Study the drawing (mm; zero at the part's minimum x, y, z) and answer. A direction names the side the tool comes from. Round coordinates to 2 decimals unless told otherwise and drop trailing zeros. Write each loop counter-clockwise with the first axis right and the second up, starting at its lowest first coordinate (ties: lowest second). Pieces come first, ordered by that corner, then holes. Notation, with made-up numbers: (66.5, -34.75) - (85.5, -34.75) arc R32 ccw to (85.5, -8.75) - close; hole circle Ø3 at (76.5, 35.5). An arc over 180 degrees is marked (long way). Use one line per item in the form item = value. Start each with the question number.
1) The part is cut by section D-D, the plane y = 35.5. Give the vertices of the cut face in (x, z), plus the area to 3 significant figures.
2) For a pull along Y with two mould halves and no side action, classify the marked faces 1, 2, 3 and 4 as released by +Y, released by -Y, zero draft, split by the parting line, or undercut.
3) The part is cut by section B-B, the plane z = 4.25. Give the vertices of the cut face in (x, y).
4) Each of these flat-tipped pins is pushed along its axis until it touches: pin 1 (1.2 mm diameter, centred on x = 15.5, z = 5, fed in from +Y); pin 2 (3 mm diameter, centred on y = 39, z = 22.5, fed in from +X); pin 3 (1.5 mm diameter, centred on x = 16.5, z = 20.5, fed in from +Y). Where does it stop, or does it pass through?
5) The part is cut by section C-C, the plane x = 11.5. Give the vertices of the cut face in (y, z), plus the area to 3 significant figures.
6) For the marked faces 5, 6, 7, 8 and 9, determine the directions among +Z, -Z, +X, -X, +Y, -Y from which every point of the face is accessible in a straight line to the end or side of a thin tool.
7) Consider line 1 along Y through (x, z) = (11, 3.2); line 2 along Z through (x, y) = (10.75, 23.5); line 3 along X through (y, z) = (26, 1.3). Determine where each line is inside the solid, lowest interval first. Write a range as from..to.
8) The part is cut by section A-A, the plane y = 6. Give the vertices of the cut face in (x, z), plus the area to 3 significant figures.
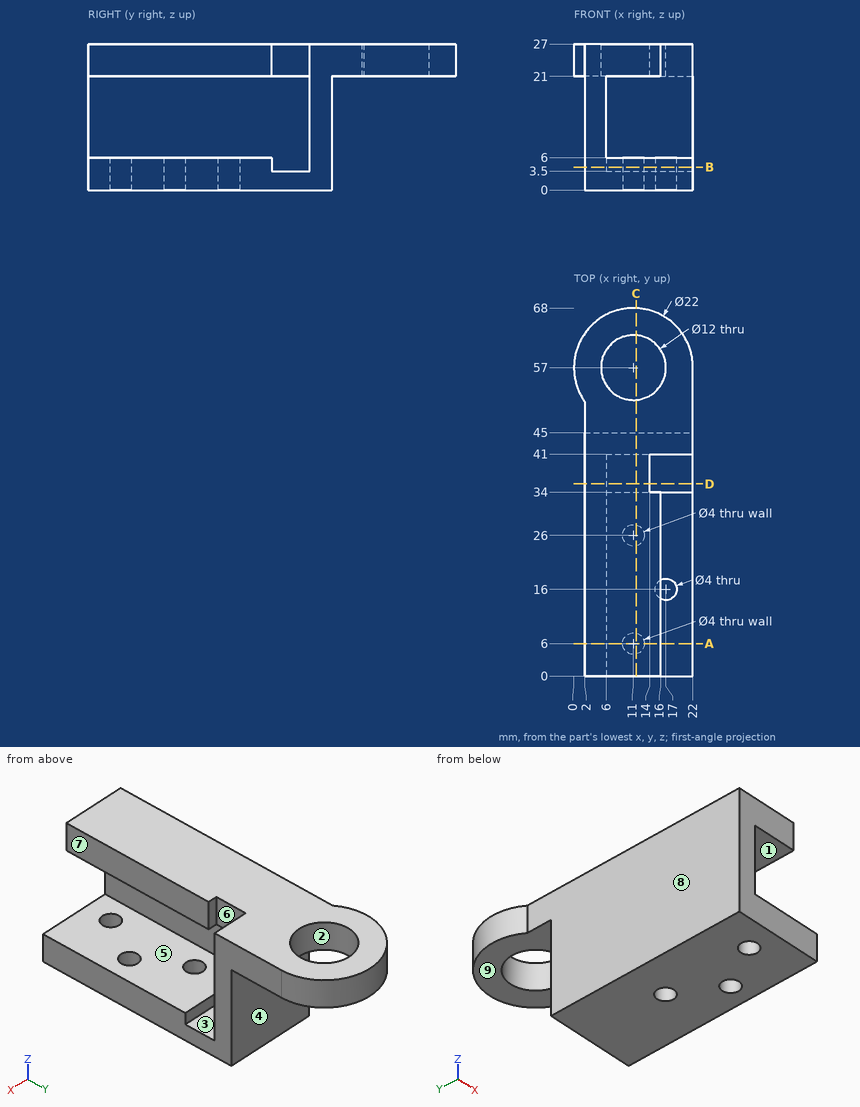
Geometry results:
q1.outline = (2, 0) - (22, 0) - (22, 3.5) - (6, 3.5) - (6, 21) - (14, 21) - (14, 27) - (2, 27) - close
q1.area = 212 mm2
q2.face_1 = zero draft
q2.face_2 = undercut
q2.face_3 = undercut
q2.face_4 = released by +Y
q3.outline = (2, 0) - (22, 0) - (22, 34) - (6, 34) - (6, 41) - (22, 41) - (22, 45) - (2, 45) - close; hole circle Ø4 at (11, 6); hole circle Ø4 at (11, 26); hole circle Ø4 at (17, 16)
q4.pin_1 = 45
q4.pin_2 = 14
q4.pin_3 = 66.83
q5.outline = (0, 0) - (4.06, 0) - (4.06, 6) - (0, 6) - close; (0, 21) - (41, 21) - (41, 3.5) - (34, 3.5) - (34, 6) - (27.94, 6) - (27.94, 0) - (45, 0) - (45, 21) - (51.02, 21) - (51.02, 27) - (0, 27) - close; (7.94, 0) - (24.06, 0) - (24.06, 6) - (7.94, 6) - close; (62.98, 21) - (67.99, 21) - (67.99, 27) - (62.98, 27) - close
q5.area = 602 mm2
q6.face_5 = +X, -Y
q6.face_6 = +Z, +X
q6.face_7 = +Z, +X, -Y
q6.face_8 = +Z, -Z, -X, -Y
q6.face_9 = -Z, +X, -X, +Y
q7.line_1 = 0..4, 8..24, 28..45
q7.line_2 = 0..6, 21..27
q7.line_3 = 2..9, 13..22
q8.outline = (2, 0) - (9, 0) - (9, 6) - (6, 6) - (6, 21) - (16, 21) - (16, 27) - (2, 27) - close; (13, 0) - (22, 0) - (22, 6) - (13, 6) - close
q8.area = 240 mm2
